Source: CAD feature listing. Evaluate the final solid. Frame: model axes, mm. Round coordinates to 2 decimals unless told otherwise and drop trailing zeros. Loops run counter-clockwise (first coordinate to the right, second up) from the corner with the lowest first, then second, coordinate; pieces in that order, holes last. Notation, with made-up numbers: M 22.5,51.5 L 72.5,51.5 A27 cw 72.5,71.5 Z; hole C 14,0 d11. An arc over 180 degrees is marked long. One line per item, written item: value.
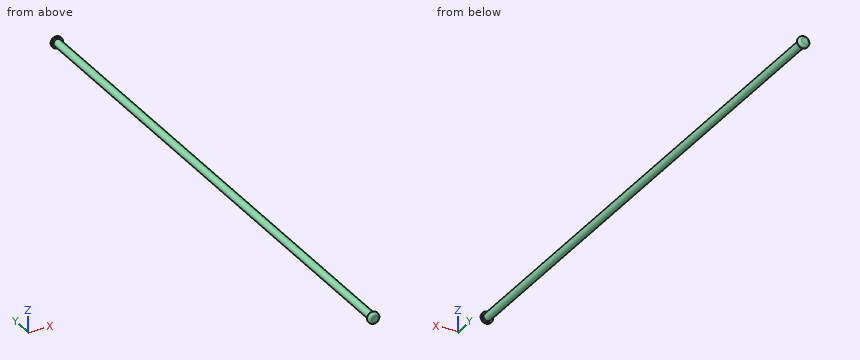
from build123d import *

# Parameters (mm, degrees)
SKETCH1_R           = 1.5
BOSS_EXTRUDE1_DEPTH = 224
SKETCH2_R           = 2.25
BOSS_EXTRUDE2_DEPTH = 1.5
FILLET1_R           = 1
BOSS_EXTRUDE3_START = -1.5
SKETCH3_R           = 2.25
BOSS_EXTRUDE3_DEPTH = 1.5
FILLET2_R           = 1


with BuildPart() as part:
    # Sketch1 → Boss-Extrude1 (new body)
    with BuildSketch(Plane(origin=(0, 0, 0), x_dir=(1, 0, 0), z_dir=(0, 1, 0))):
        with Locations(Location((0, 0, 0), (0, 0, 270))):
            Circle(SKETCH1_R)
    extrude(amount=BOSS_EXTRUDE1_DEPTH)

    # Sketch2 → Boss-Extrude2 (add)
    with BuildSketch(Plane(origin=(0, 224, 0), x_dir=(1, 0, 0), z_dir=(0, 1, 0))):
        with Locations(Location((0, 0, 0), (0, 0, 270))):
            Circle(SKETCH2_R)
    extrude(amount=-BOSS_EXTRUDE2_DEPTH)

    # Fillet1
    fillet1_edges = [part.edges().sort_by_distance(p)[0] for p in [
        (0, 224, -2.25),
    ]]
    fillet(fillet1_edges, radius=FILLET1_R)

    # Sketch3 → Boss-Extrude3 (add)
    with BuildSketch(Plane.XZ.offset(BOSS_EXTRUDE3_START)):
        with Locations(Location((0, 0, 0), (0, 0, 90))):
            Circle(SKETCH3_R)
    extrude(amount=BOSS_EXTRUDE3_DEPTH)

    # Fillet2
    fillet2_edges = [part.edges().sort_by_distance(p)[0] for p in [
        (0, 0, -2.25),
    ]]
    fillet(fillet2_edges, radius=FILLET2_R)


solid = part.part
1. Section query B-B (x = 0). Return the cut outline in (y, z), and give its area (3 significant figures).
Report:
outline: M 0,-1.25 A1 ccw 1,-2.25 L 1.5,-2.25 L 1.5,-1.5 L 222.5,-1.5 L 222.5,-2.25 L 223,-2.25 A1 ccw 224,-1.25 L 224,1.25 A1 ccw 223,2.25 L 222.5,2.25 L 222.5,1.5 L 1.5,1.5 L 1.5,2.25 L 1,2.25 A1 ccw 0,1.25 Z
area: 676 mm2
2. Pin query (flat end, axial travel): pin 1 (1.5 mm diameter, centred on x = -1.5, z = -1.5, fed in from +Y); pin 2 (2 mm diameter, centred on x = 1.5, y = 100, fed in from -Z). Return the tip coordinate at first contact, or that it passes through.
Report:
pin 1: stops at y = 223.99
pin 2: stops at z = -1.41
3. Section query C-C (y = 25). Return the cut outline in (x, z).
Report:
outline: C 0,0 d3
4. Section query A-A (z = 0). Return the cut outline in (x, y), and give its area (3 significant figures).
Report:
outline: M -2.25,1 A1 ccw -1.25,0 L 1.25,0 A1 ccw 2.25,1 L 2.25,1.5 L 1.5,1.5 L 1.5,222.5 L 2.25,222.5 L 2.25,223 A1 ccw 1.25,224 L -1.25,224 A1 ccw -2.25,223 L -2.25,222.5 L -1.5,222.5 L -1.5,1.5 L -2.25,1.5 Z
area: 676 mm2
5. Ray query, line 1 (X direction, y = 152.5, z = 0.2); line 2 (Z direction, x = 0, y = 38); line 3 (Y direction, x = 0.5, z = -1.25). Return the intervals inside material, ascending. Write a range as [from, to].
Report:
line 1: x = [-1.49, 1.49]
line 2: z = [-1.5, 1.5]
line 3: y = [0, 224]
